The figure shows three views and two pictorial views of one solid part (mm, origin at its lowest corner). Answer the questions. A direction names the side the tool comes from. Coordinates: 2 decimals unless noted, no trailing zeros. Loops run counter-clockwise (first coordinate to the right, second up) from the corner with the lowest first, then second, coordinate; pieces in that order, holes last. Notation, with made-up numbers: M -4,-34 L 44,-34 A27 cw 44,-9 Z; hole C 64.5,79.5 d3. An arc over 180 degrees is marked long. Write each question's results on one line, items separated by ' | '.
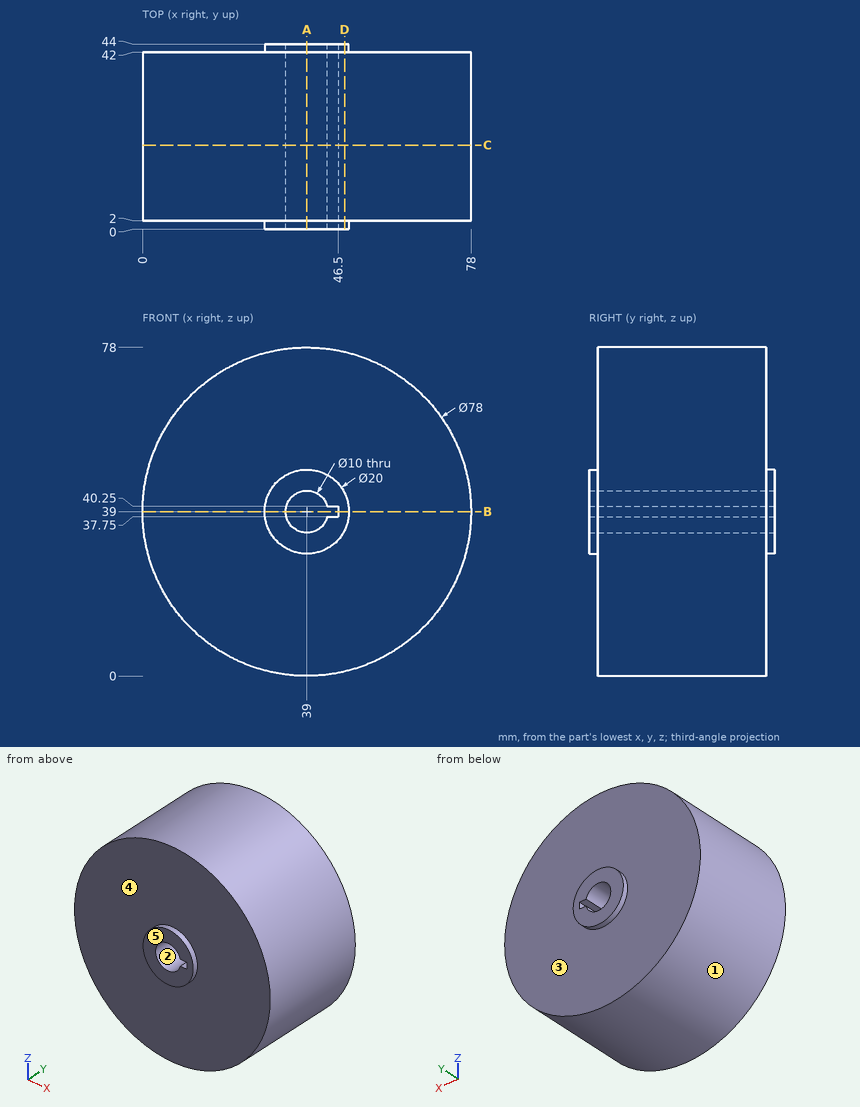
1) Straight lines are drawn through the part: probe 1 along X at (y, z) = (29, 39); probe 2 along Z at (x, y) = (39, 23.5); probe 3 along Y at (x, z) = (64, 68). For each, find the intervals that lie inside material, in ascending order. Write a range as [from, to].
Check result:
probe 1: [0, 34], [46.5, 78] | probe 2: [0, 34], [44, 78] | probe 3: [2, 42]
2) For a pull along Z with two mould halves and no side action, classify the marked faces 1, 2 and 3 as released by +Z, released by -Z, zero draft, split by the parting line, or undercut.
Check result:
face 1: split by the parting line | face 2: undercut | face 3: zero draft
3) Given pin 1 Ø4 at (y, z) = (36, 27) entering from -X; pin 2 Ø0.8 at (x, y) = (45, 21) entering from +Z; pin 3 Ø1.5 at (x, z) = (57.5, 61.5) entering from -Y, each flat-ended and moving along its own axis, determine where each tip first touches the part or whether it passes through.
Check result:
pin 1: x = 1.3 | pin 2: z = 77.6 | pin 3: y = 2
4) Find section A-A, the plane x = 39. Give the vertices of the cut face in (y, z).
Check result:
outline: M 0,29 L 2,29 L 2,0 L 42,0 L 42,29 L 44,29 L 44,34 L 0,34 Z; M 0,44 L 44,44 L 44,49 L 42,49 L 42,78 L 2,78 L 2,49 L 0,49 Z
5) Find section C-C, the plane y = 20. Give the vertices of the cut face in (x, z).
Check result:
outline: C 39,39 d78; hole M 43.84,37.75 L 46.5,37.75 L 46.5,40.25 L 43.84,40.25 A5 ccw long Z
6) Find section B-B, the plane z = 39. Give the vertices of the cut face in (x, y), and give its area (3 significant figures).
Check result:
outline: M 0,2 L 29,2 L 29,0 L 34,0 L 34,44 L 29,44 L 29,42 L 0,42 Z; M 46.5,0 L 49,0 L 49,2 L 78,2 L 78,42 L 49,42 L 49,44 L 46.5,44 Z | area: 2,650 mm^2
7) Which of the six approach directions +Z, -Z, +X, -X, +Y, -Y give full straight-line access (tool end or side, diameter ignored) to the marked faces 4 and 5?
Check result:
face 4: -Y | face 5: +Z, -Z, +X, -X, -Y
8) Find section D-D, the plane x = 48. Give the vertices of the cut face in (y, z).
Check result:
outline: M 0,34.64 L 2,34.64 L 2,1.05 L 42,1.05 L 42,34.64 L 44,34.64 L 44,43.36 L 42,43.36 L 42,76.95 L 2,76.95 L 2,43.36 L 0,43.36 Z
